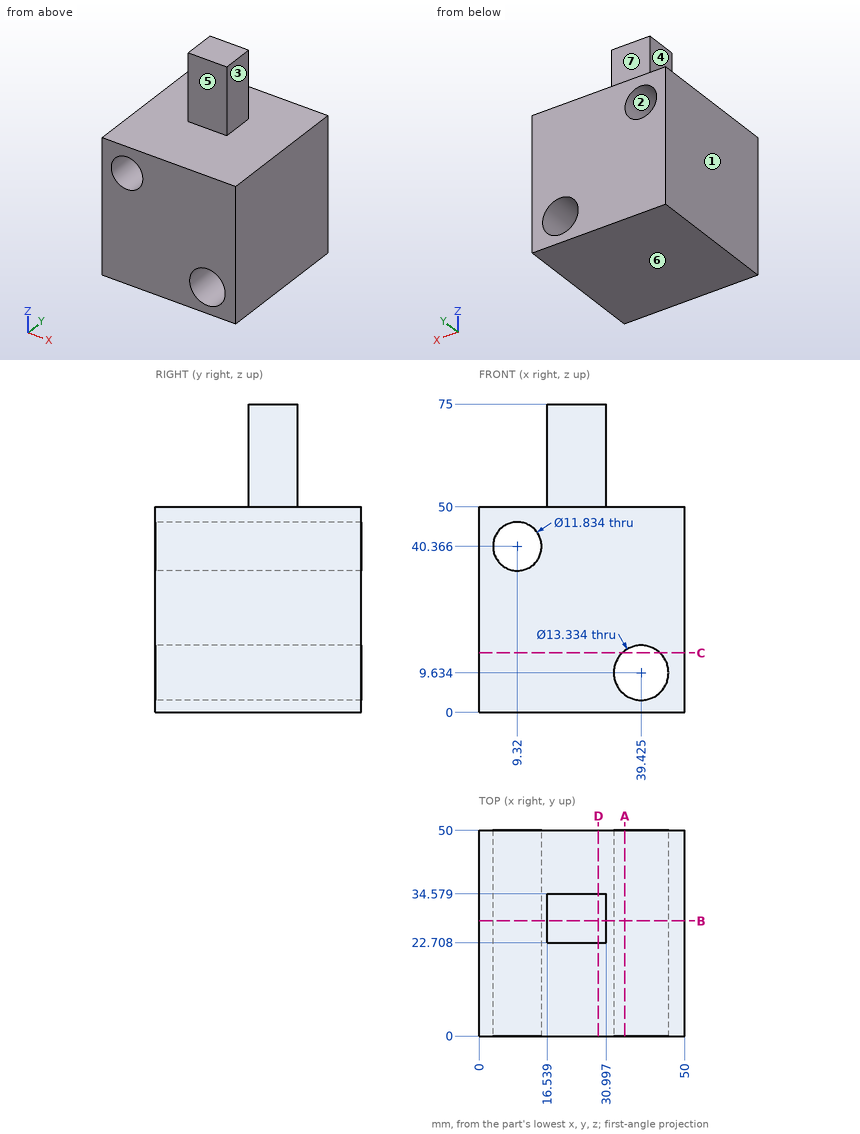
Check sheet for the drawn part. Datum: minimum x, y, z corner. Units: mm. A direction names the side the tool comes from. Round coordinates to 2 decimals unless told otherwise and drop trailing zeros. Loops run counter-clockwise (first coordinate to the right, second up) from the corner with the lowest first, then second, coordinate; pieces in that order, holes last.
Item 1: Cross-section at B-B on y = 28. Record the boundary of the cut face in (x, z) (1 decimal), then the cut area to 3 significant figures.
Item 2: Cross-section at A-A on x = 35.5. Record the boundary of the cut face in (y, z) (1 decimal), then the cut area to 3 significant figures.
Item 3: Thickness scan on line 1 (Z direction, x = 39, y = 44); line 2 (X direction, y = 16, z = 39); line 3 (X direction, y = 33, z = 7). Record the ranges inside material, lowest first.
Item 4: Gauge pin test, flat ends, axial feed: pin 1 (10 mm diameter, centred on x = 14.5, z = 65.5, fed in from -Y); pin 2 (3.5 mm diameter, centred on y = 29, z = 62.5, fed in from +X); pin 3 (4.5 mm diameter, centred on x = 27, z = 68, fed in from +Y); pin 4 (6 mm diameter, centred on y = 12.5, z = 54.5, fed in from -X). Record the tip position at first contact, or that the pin passes through.
Item 5: Cross-section at C-C on z = 14.5. Record the boundary of the cut face in (x, y), then the cut area to 3 significant figures.
Item 6: Cross-section at D-D on x = 29. Record the boundary of the cut face in (y, z), then the cut area to 3 significant figures.
Item 7: Mould release check, pull along X, two halves, no side actions. Record for the marked faces 1, 2 and 3: pulls with the +X half, pulls with the -X half, needs draft (parallel to the pull), parting line crosses it, or undercut.
Item 8: Access from +Z, -Z, +X, -X, +Y, -Y to the whole of each face (thin tool, end or side, straight path). Record for the marked faces 4, 5, 6 and 7.
Answer sheet:
1. outline: (0, 0) - (50, 0) - (50, 50) - (31, 50) - (31, 75) - (16.5, 75) - (16.5, 50) - (0, 50) - close; hole circle Ø11.8 at (9.3, 40.4); hole circle Ø13.3 at (39.4, 9.6)
1. area: 2,610 mm2
2. outline: (0, 0) - (50, 0) - (50, 4.2) - (0, 4.2) - close; (0, 15) - (50, 15) - (50, 50) - (0, 50) - close
2. area: 1,960 mm2
3. line 1: z = 0 to 2.98, 16.29 to 50
3. line 2: x = 0 to 3.56, 15.08 to 50
3. line 3: x = 0 to 33.3, 45.55 to 50
4. pin 1: stops at y = 22.71
4. pin 2: stops at x = 31
4. pin 3: stops at y = 34.58
4. pin 4: passes through
5. outline: (0, 0) - (34.87, 0) - (34.87, 50) - (0, 50) - close; (43.98, 0) - (50, 0) - (50, 50) - (43.98, 50) - close
5. area: 2,040 mm2
6. outline: (0, 0) - (50, 0) - (50, 50) - (34.58, 50) - (34.58, 75) - (22.71, 75) - (22.71, 50) - (0, 50) - close
6. area: 2,800 mm2
7. face 1: pulls with the -X half
7. face 2: undercut
7. face 3: pulls with the +X half
8. face 4: +Z, -X, +Y, -Y
8. face 5: +Z, +X, -X, -Y
8. face 6: -Z, +X, -X, +Y, -Y
8. face 7: +Z, +X, -X, +Y
